Could you check a few things on this model? Use its own coordinates, in mm. Face numbers are marked on the shaded views. A direction names the side the tool comes from. Coordinates: 2 decimals unless noted, no trailing zeros. Write each loop counter-clockwise with the first axis right and the second up, starting at its lowest first coordinate (ties: lowest second). Pieces come first, ordered by that corner, then holes.
```python
from build123d import *

# Parameters (mm, degrees)
EXTRUDE_1_DEPTH      = 6
SKETCH_23_W          = 7
SKETCH_23_H          = 6
EXTRUDE_23_DEPTH     = 6
CUT_EXTRUDE_11_DEPTH = 7
SKETCH_2_W           = 7
SKETCH_2_H           = 6
EXTRUDE_2_DEPTH      = 6
CUT_EXTRUDE_1_DEPTH  = 7
SKETCH_24_W          = 7
SKETCH_24_H          = 6
EXTRUDE_24_DEPTH     = 6
SKETCH_25_W          = 7
SKETCH_25_H          = 6
EXTRUDE_26_DEPTH     = 6


with BuildPart() as part:
    # Эскиз1 → Бобышка-Вытянуть1 (new body)
    with BuildSketch(Plane.XY):
        with BuildLine():
            Line((47, 6.078379342), (6, 6.078379342))
            Line((6, 6.078379342), (6, 40.147643713))
            Line((6, 40.147643713), (9.160917848, 40.103855916))
            ThreePointArc((9.160917848, 40.103855916), (10.882668259, 39.772556875), (12.384183162, 38.867219076))
            Line((12.384183162, 38.867219076), (45.292523039, 10.072421683))
            ThreePointArc((45.292523039, 10.072421683), (46.55316457, 8.375619622), (47, 6.309538209))
            Line((47, 6.309538209), (47, 6.078379342))
        make_face()
    extrude(amount=-EXTRUDE_1_DEPTH)

    # Эскиз23 → Бобышка-Вытянуть23 (add)
    with BuildSketch(Plane(origin=(27, 56.078379342, -6), x_dir=(1, 0, 0), z_dir=(0, 0, -1))):
        with Locations((-9.531849908, 53)):
            Rectangle(SKETCH_23_W, SKETCH_23_H)
        with Locations((9.531849908, 53)):
            Rectangle(SKETCH_23_W, SKETCH_23_H)
    extrude(amount=-EXTRUDE_23_DEPTH)

    # Эскиз31 → Вырез-Вытянуть11 (cut, through all)
    with BuildSketch(Plane(origin=(27, 56.078379342, -6), x_dir=(1, 0, 0), z_dir=(0, 0, -1))):
        Polygon((-2.1, 45), (-3.6, 45), (-3.6, 42.6), (-2.1, 42.6), (-2.1, 37.5), (2.1, 37.5), (2.1, 42.6), (3.6, 42.6), (3.6, 45), (2.1, 45), (2.1, 50), (-2.1, 50), align=None)
    extrude(amount=-CUT_EXTRUDE_11_DEPTH, mode=Mode.SUBTRACT)

    # Эскиз2 → Бобышка-Вытянуть2 (add)
    with BuildSketch(Plane(origin=(56, 23.078379342, -6), x_dir=(0, -1, 0), z_dir=(0, 0, -1))):
        with Locations((-9.531849908, 53)):
            Rectangle(SKETCH_2_W, SKETCH_2_H)
        with Locations((9.531849908, 53)):
            Rectangle(SKETCH_2_W, SKETCH_2_H)
    extrude(amount=-EXTRUDE_2_DEPTH)

    # Эскиз3 → Вырез-Вытянуть1 (cut, through all)
    with BuildSketch(Plane(origin=(56, 23.078379342, -6), x_dir=(0, -1, 0), z_dir=(0, 0, -1))):
        Polygon((-2.1, 45), (-3.6, 45), (-3.6, 42.6), (-2.1, 42.6), (-2.1, 39), (2.1, 39), (2.1, 42.6), (3.6, 42.6), (3.6, 45), (2.1, 45), (2.1, 50), (-2.1, 50), align=None)
    extrude(amount=-CUT_EXTRUDE_1_DEPTH, mode=Mode.SUBTRACT)

    # Эскиз24 → Бобышка-Вытянуть24 (add)
    with BuildSketch(Plane(origin=(56, 23.078379342, 0), x_dir=(0, 1, 0), z_dir=(0, 0, 1))):
        with Locations((-9.531849908, 53)):
            Rectangle(SKETCH_24_W, SKETCH_24_H)
        with Locations((9.531849908, 53)):
            Rectangle(SKETCH_24_W, SKETCH_24_H)
    extrude(amount=-EXTRUDE_24_DEPTH)

    # Эскиз25 → Бобышка-Вытянуть26 (add)
    with BuildSketch(Plane(origin=(27, 56.078379342, -6), x_dir=(1, 0, 0), z_dir=(0, 0, -1))):
        with Locations((-9.531849908, 53)):
            Rectangle(SKETCH_25_W, SKETCH_25_H)
        with Locations((9.531849908, 53)):
            Rectangle(SKETCH_25_W, SKETCH_25_H)
    extrude(amount=-EXTRUDE_26_DEPTH)


solid = part.part
```
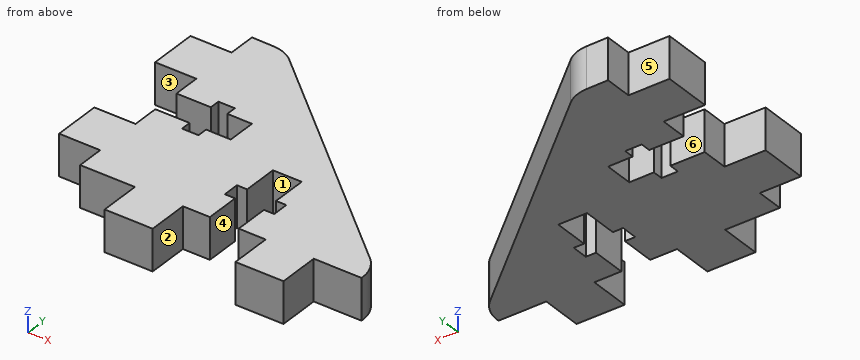
1. I want a section at C-C on x = 28.5. Please give me the cut outline in (y, z).
Verdict:
outline: (18.58, -6) - (24.77, -6) - (24.77, 0) - (18.58, 0) - close
2. I want a section at D-D on x = 22. Please give me the cut outline in (y, z), plus the area to 3 significant figures.
Verdict:
outline: (6.08, -6) - (30.45, -6) - (30.45, 0) - (6.08, 0) - close
area: 146 mm2
3. For pin 1 (0.8 mm diameter, centred on y = 26, z = -2, fed in from +X); pin 2 (2.5 mm diameter, centred on y = 8, z = -3.5, fed in from -X); pin 3 (0.7 mm diameter, centred on x = 12.5, z = -4.5, fed in from +Y), each with a flat end and sliding along its axis, tell me the tip position at first contact or that it passes through.
Verdict:
pin 1: stops at x = 27.55
pin 2: stops at x = 6
pin 3: stops at y = 39.06
4. On a 3-axis mill with a long thin cutter (end or side, diameter ignored), from which of +Z, -Z, +X, -X, +Y, -Y can I reach the whole of each face in a straight line? I mean the marked faces 4, 5 and 6. Say none if no direction works.
Verdict:
face 4: +Z, -Z, -Y
face 5: +Z, -Z, -X, +Y
face 6: +Z, -Z, -X
5. I want a section at A-A on x = 7. Please give me the cut outline in (y, z).
Verdict:
outline: (6.08, -6) - (20.98, -6) - (20.98, 0) - (6.08, 0) - close; (25.18, -6) - (40.13, -6) - (40.13, 0) - (25.18, 0) - close
6. Please list where these lines run through material, in increasing order: line 1 along X through (y, z) = (11, -3.45); line 2 along Y through (x, z) = (24, -3.45); line 3 along X through (y, z) = (8, -2.4).
Verdict:
line 1: x = 0 to 24.9, 29.1 to 44.23
line 2: y = 6.08 to 11.08, 13.48 to 28.7
line 3: x = 6 to 24.9, 29.1 to 46.71
7. If we mould it in two halves opening along Y, with no side actions, what happens to the marked faces 1, 2 and 3? For each: pulls with the +Y half, pulls with the -Y half, needs draft (parallel to the pull), parting line crosses it, or undercut.
Verdict:
face 1: pulls with the -Y half
face 2: needs draft
face 3: undercut
8. I want a section at B-B on y = 16. Please give me the cut outline in (x, z), plus the area to 3 significant figures.
Verdict:
outline: (0, -6) - (24.9, -6) - (24.9, 0) - (0, 0) - close; (29.1, -6) - (38.52, -6) - (38.52, 0) - (29.1, 0) - close
area: 206 mm2
